```python
from build123d import *

# Parameters (mm, degrees)
F0_W     = 101.6
F0_H     = 60
F1_DEPTH = 19.05
F2_R     = 9.525
F3_DEPTH = 6.35
F5_DEPTH = 10


# Not quite as in the source:
# - a length typed as a fraction of an inch, garbled in the dataset ("3 / 203.2 mm" for 3/8 in), is restored


with BuildPart() as f1:
    # F0 (on Top) → F1 (new body)
    with BuildSketch(Plane.XY):
        Rectangle(F0_W, F0_H)
    extrude(amount=F1_DEPTH)

    # F2 (on face) → F3 (cut)
    with BuildSketch(Plane.XY.offset(19.05)):
        Circle(F2_R)
        with Locations((31.75, 0)):
            Circle(F2_R)
        with Locations((-31.75, 0)):
            Circle(F2_R)
    extrude(amount=-F3_DEPTH, mode=Mode.SUBTRACT)

    # F4 (on face) → F5 (join)
    with BuildSketch(Plane(origin=(0, 30, 0), x_dir=(-1, 0, 0), z_dir=(0, 1, 0))):
        with BuildLine():
            ThreePointArc((-12.7, 0), (-25.4, 12.7), (-38.1, 0))
            Line((-38.1, 0), (-25.4, 0))
            Line((-25.4, 0), (-12.7, 0))
        make_face()
        with BuildLine():
            Line((-25.4, 0), (-38.1, 0))
            ThreePointArc((-38.1, 0), (-25.4, -12.7), (-12.7, 0))
            Line((-12.7, 0), (-25.4, 0))
        make_face()
    extrude(amount=F5_DEPTH)


with BuildPart() as f6_1:
    # F6: instance of F1
    add(f1.part.mirror(Plane.YZ))


with BuildPart() as f1_1:
    add(f1.part)

    add(f6_1.part)  # F7 merges F6_1
    # F7: F6_1, F1 across plane
    add(f6_1.part.mirror(Plane.XZ))
    add(f1.part.mirror(Plane.XZ))


solid = f1_1.part
```
Geometry: final body of the model. Coordinates: model frame, mm. A direction names the side the tool comes from. Coordinates: 2 decimals unless noted, no trailing zeros. Write each loop counter-clockwise with the first axis right and the second up, starting at its lowest first coordinate (ties: lowest second). Pieces come first, ordered by that corner, then holes. Notation, with made-up numbers: M 54.5,43 L 58.5,43 A26 cw 58.5,60 Z; hole C 88,-5.5 d8. An arc over 180 degrees is marked long. Answer as CSV lines item,"result". Start each with the question number.
Q1. Cut plane C-C on z = -10. Return the cut outline in (x, y).
Q2. Cut plane D-D on y = -32.5. Return the cut outline in (x, z).
Q3. Line query: line 1 (X direction, y = 0, z = 14) (3 decimals); line 2 (Y direction, x = 31.75, z = 14) (3 decimals); line 3 (X direction, y = 1, z = 16). Output: solid intervals per line, ascending. Write a range as from..to.
Q4. Pin query (flat end, axial travel): P1, Ø6, axis at x = 9, y = -18, coming from the -Z side; P2, Ø8, axis at y = 31, z = -9, coming from the -X side. Return the tip coordinate at first contact, or that it passes through.
Q5. Cut plane B-B on x = 0. Return the cut outline in (y, z) (3 decimals).
Q6. Mould query, pull axis Y, two halves, no side actions, for faces 1 (the flat face through (26, -30, -5)), 2 (the flat face through (-50.8, 0, 9)), 3 (the flat face through (-26, 40, 0)). Classes: released by +Y, released by -Y, zero draft, split by the parting line, or undercut.
Q7. Cut plane A-A on z = 17. Return the cut outline in (x, y) (3 decimals), then the cut area to 3 significant figures.
Q8. Reachability of faces 4 (the flat face through (-32, 0, 12.7)), 5 (the flat face through (26, 30, -5)), 6 (the cylindrical face through (12.712, -34.93, -0.558)), 7 (the cylindrical face through (12.712, 34.93, -0.558)) from +Z, -Z, +X, -X, +Y, -Y: full face, straight path, thin tool, end or side. Return the list, or none.
Findings below:
1,outline,"M -33.23,-40 L -17.57,-40 L -17.57,-30 L -33.23,-30 Z; M -33.23,30 L -17.57,30 L -17.57,40 L -33.23,40 Z; M 17.57,-40 L 33.23,-40 L 33.23,-30 L 17.57,-30 Z; M 17.57,30 L 33.23,30 L 33.23,40 L 17.57,40 Z"
2,outline,"C -25.4,0 d25.4; C 25.4,0 d25.4"
3,line 1,"x = -50.8..-41.275, -22.225..-9.525, 9.525..22.225, 41.275..50.8"
3,line 2,"y = -30..-9.525, 9.525..30"
3,line 3,"x = -50.8..-41.22, -22.28..-9.47, 9.47..22.28, 41.22..50.8"
4,P1,"stops at z = 0"
4,P2,"stops at x = -37.07"
5,outline,"M -30,0 L 30,0 L 30,19.05 L 9.525,19.05 L 9.525,12.7 L -9.525,12.7 L -9.525,19.05 L -30,19.05 Z"
6,face 1,"undercut"
6,face 2,"zero draft"
6,face 3,"released by +Y"
7,outline,"M -50.8,-30 L 50.8,-30 L 50.8,30 L -50.8,30 Z; hole C -31.75,0 d19.05; hole C 0,0 d19.05; hole C 31.75,0 d19.05"
7,area,"5,240 mm2"
8,face 4,"+Z"
8,face 5,"-Z, +X, -X"
8,face 6,"-Y"
8,face 7,"+Y"
